Build history of the part. All positions in model axes, mm. A direction names the side the tool comes from. Round coordinates to 2 decimals unless told otherwise and drop trailing zeros. Order: outer loops, then holes, each group sorted by start corner. A loop starts at its lowest first (then second) coordinate and runs counter-clockwise, first axis right, second up. Notation, with made-up numbers: (-26.5, 32) -> (25.5, 32) arc R27 cw to (25.5, 68) -> close; hole circle Ø8 at (38, -19.75). An arc over 180 degrees is marked (long way). Write item = value, one per line.
from build123d import *

# Parameters (mm, degrees)
F0_R     = 6.5
F1_DEPTH = 13
F2_R     = 3
F3_DEPTH = 21.5
F4_R     = 3
F5_DEPTH = 19
F7_D     = 11


with BuildPart() as f1:
    # F0 (on Top) → F1 (new body)
    with BuildSketch(Plane.XY):
        Circle(F0_R)
    extrude(amount=F1_DEPTH)

    # F2 (on Right) → F3 (join, symmetric)
    with BuildSketch(Plane.YZ):
        with Locations((0, 8)):
            Circle(F2_R)
    extrude(amount=F3_DEPTH, both=True)

    # F4 (on Front) → F5 (join)
    with BuildSketch(Plane.XZ):
        with Locations((0, 8)):
            Circle(F4_R)
    extrude(amount=F5_DEPTH)

    # F7 (through all)
    with Locations(Plane(origin=(0, 0, 0), x_dir=(1, 0, 0), z_dir=(0, 0, -1))):
        with Locations((0, 0)):
            Hole(F7_D / 2)


solid = f1.part
Q1. Probe probe 1 along Y at (x, z) = (0, 6.25); probe 2 along Y at (x, z) = (-7, 7.75); probe 3 along X at (y, z) = (0.5, 3.75). List the from-to ranges inside material, lowest first.
Check values:
probe_1 = -19 to -5.5, 5.5 to 6.5
probe_2 = -2.99 to 2.99
probe_3 = -6.48 to -5.48, 5.48 to 6.48
Q2. Mould opens along Y. For faces 4 (the face through (13.74, 1.61, 10.53)), 5 (the face through (-21.5, 0, 8)), 6 (the face through (1.19, 5.37, 6.59)) say: released by +Y, released by -Y, zero draft, split by the parting line, or undercut.
Check values:
face_4 = split by the parting line
face_5 = zero draft
face_6 = undercut
Q3. Cut at A-A, the plane y = 0. List the corners of the cut face in (x, z).
Check values:
outline = (-21.5, 5) -> (-6.5, 5) -> (-6.5, 0) -> (-5.5, 0) -> (-5.5, 13) -> (-6.5, 13) -> (-6.5, 11) -> (-21.5, 11) -> close; (5.5, 0) -> (6.5, 0) -> (6.5, 5) -> (21.5, 5) -> (21.5, 11) -> (6.5, 11) -> (6.5, 13) -> (5.5, 13) -> close
Q4. Cut at D-D, the plane x = 12.5. List the corners of the cut face in (y, z), and give its area (3 significant figures).
Check values:
outline = circle Ø6 at (0, 8)
area = 28.3 mm²
Q5. Cut at C-C, the plane z = 10.5. List the corners of the cut face in (x, y).
Check values:
outline = (-21.5, -1.66) -> (-6.28, -1.66) arc R6.5 ccw to (-1.66, -6.28) -> (-1.66, -19) -> (1.66, -19) -> (1.66, -6.28) arc R6.5 ccw to (6.28, -1.66) -> (21.5, -1.66) -> (21.5, 1.66) -> (6.28, 1.66) arc R6.5 ccw to (-6.28, 1.66) -> (-21.5, 1.66) -> close; hole circle Ø11 at (0, 0)
Q6. Which spindle directions (+Z, -Z, +X, -X, +Y, -Y) get a long thin tool onto all of the face, cutting with end or side? Do faces 1 (the face through (21.5, 0, 8)), 2 (the face through (-13.52, 1.61, 10.53)), 3 (the face through (2.86, -12.29, 8.9)). Say none if no direction does.
Check values:
face_1 = +Z, -Z, +X, +Y, -Y
face_2 = -X
face_3 = -Y
Q7. Cut at B-B, the plane x = 0. List the corners of the cut face in (y, z).
Check values:
outline = (-19, 5) -> (-6.5, 5) -> (-6.5, 0) -> (-5.5, 0) -> (-5.5, 13) -> (-6.5, 13) -> (-6.5, 11) -> (-19, 11) -> close; (5.5, 0) -> (6.5, 0) -> (6.5, 13) -> (5.5, 13) -> close
Q8. Flat gauge pins, fed straight in: pin 1 (6 mm diameter, centred on y = -12, z = 8, fed in from +X); pin 2 (3 mm diameter, centred on x = -2.5, y = -15.5, fed in from -Z); pin 3 (4 mm diameter, centred on y = -12, z = 11, fed in from -X). Where does each tip first touch, or does it go through?
Check values:
pin_1 = 3
pin_2 = 5.17
pin_3 = -2.83
